Part print with two shaded views. Sizes in mm from the minimum x, y, z corner. A direction names the side the tool comes from. Coordinates: 2 decimals unless noted, no trailing zeros. Loops run counter-clockwise (first coordinate to the right, second up) from the corner with the lowest first, then second, coordinate; pieces in that order, holes last.
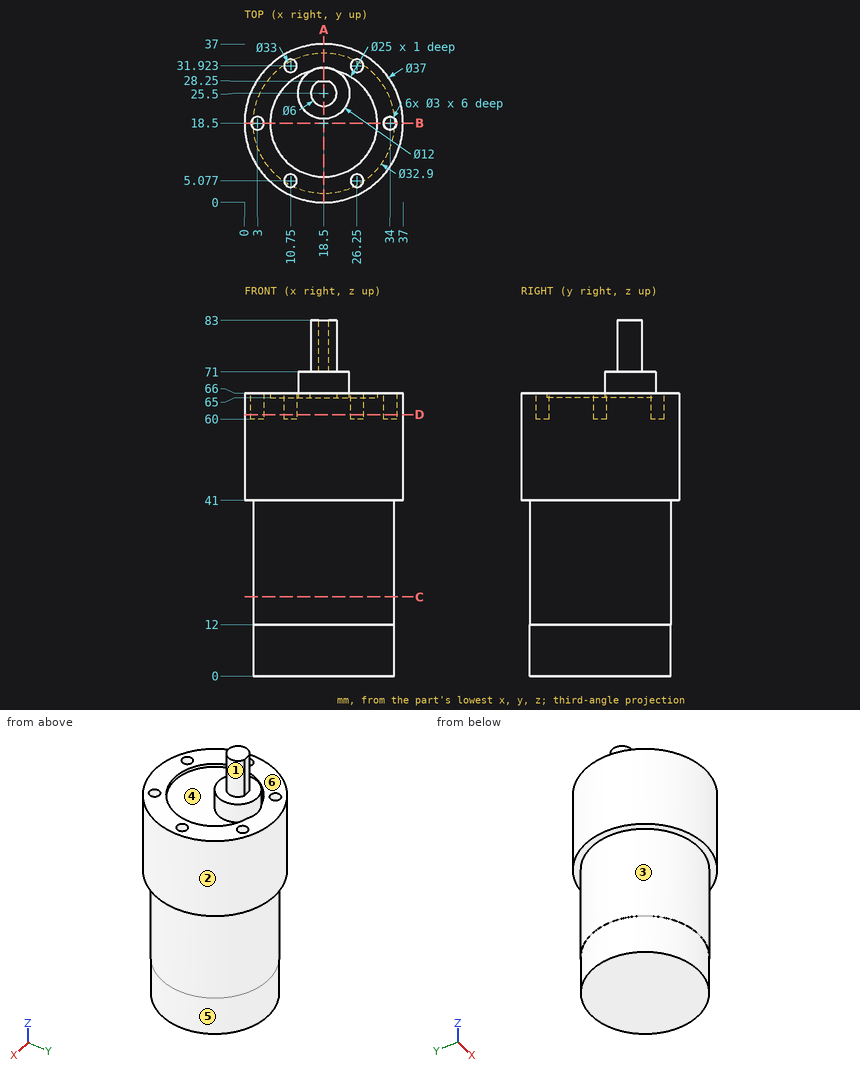
Q1. Slice it at B-B (y = 18.5). List the corners of the cut face in (x, z), and give its area (3 significant figures).
Answers:
outline: (0, 41) - (2, 41) - (2, 12) - (2.05, 12) - (2.05, 0) - (34.95, 0) - (34.95, 12) - (35, 12) - (35, 41) - (37, 41) - (37, 66) - (35.5, 66) - (35.5, 60) - (32.5, 60) - (32.5, 66) - (31, 66) - (31, 65) - (6, 65) - (6, 66) - (4.5, 66) - (4.5, 60) - (1.5, 60) - (1.5, 66) - (0, 66) - close
area: 2,220 mm2
Q2. Drill centre lines: line 1 (Y direction, x = 26.25, z = 64.1); line 2 (Z direction, x = 7, y = 26); line 3 (Y direction, x = 34, z = 64). Where is each one in solid material? Low to high.
Answers:
line 1: y = 1.7 to 3.58, 6.58 to 30.42, 33.42 to 35.3
line 2: z = 0 to 66
line 3: y = 8.4 to 17, 20 to 28.6
Q3. Flat gauge pins, fed straight in: P1, Ø1.5, axis at y = 5.5, z = 23.5, coming from the -X side (1 decimal); P2, Ø0.9, axis at x = 10.5, y = 32.5, coming from the +Z side; P3, Ø2.5, axis at x = 3, y = 18, coming from the +Z side. Where does each tip first touch, or does it go through?
Answers:
P1: stops at x = 7.4
P2: stops at z = 60
P3: stops at z = 66
Q4. Slice it at C-C (z = 18.5). List the corners of the cut face in (x, y), and give its area (3 significant figures).
Answers:
outline: circle Ø33 at (18.5, 18.5)
area: 855 mm2
Q5. Slice it at A-A (x = 18.5). List the corners of the cut face in (y, z).
Answers:
outline: (0, 41) - (2, 41) - (2, 12) - (2.05, 12) - (2.05, 0) - (34.95, 0) - (34.95, 12) - (35, 12) - (35, 41) - (37, 41) - (37, 66) - (31.5, 66) - (31.5, 71) - (28.25, 71) - (28.25, 83) - (22.5, 83) - (22.5, 71) - (19.5, 71) - (19.5, 65) - (6, 65) - (6, 66) - (0, 66) - close
Q6. Mould opens along Y. For the marked faces 4, 5 and 6 say: +Y half, -Y half, draft (parallel to the pull), parting line (faces both ways), or undercut.
Answers:
face 4: undercut
face 5: parting line
face 6: draft
Q7. Which spindle directions (+Z, -Z, +X, -X, +Y, -Y) get a long thin tool onto all of the face, cutting with end or side? Do the marked faces 1, 2 and 3. Say none if no direction does.
Answers:
face 1: +Z
face 2: +Z, -Z
face 3: -Z
Q8. Slice it at D-D (z = 61). List the corners of the cut face in (x, y), and give its area (3 significant figures).
Answers:
outline: circle Ø37 at (18.5, 18.5); hole circle Ø3 at (3, 18.5); hole circle Ø3 at (10.75, 5.08); hole circle Ø3 at (10.75, 31.92); hole circle Ø3 at (26.25, 5.08); hole circle Ø3 at (26.25, 31.92); hole circle Ø3 at (34, 18.5)
area: 1,030 mm2
